```python
from build123d import *

# Parameters (mm, degrees)
ESQUISSE1_R        = 13
BOSS_EXTRU_1_DEPTH = 6.9
ESQUISSE2_R        = 3
BOSS_EXTRU_2_DEPTH = 1
ESQUISSE3_R        = 0.75
BOSS_EXTRU_3_DEPTH = 6
BOSS_EXTRU_4_START = 2.3
ESQUISSE4_R        = 3
BOSS_EXTRU_4_DEPTH = 2.3


with BuildPart() as part:
    # Esquisse1 → Boss.-Extru.1 (new body)
    with BuildSketch(Plane.XY):
        with Locations(Location((0, 0, 0), (0, 0, 180))):
            Circle(ESQUISSE1_R)
    extrude(amount=BOSS_EXTRU_1_DEPTH)

    # Esquisse2 → Boss.-Extru.2 (add)
    with BuildSketch(Plane.XY.offset(6.9)):
        Circle(ESQUISSE2_R)
    extrude(amount=BOSS_EXTRU_2_DEPTH)

    # Esquisse3 → Boss.-Extru.3 (add)
    with BuildSketch(Plane.XY.offset(7.9)):
        Circle(ESQUISSE3_R)
    extrude(amount=BOSS_EXTRU_3_DEPTH)

    # Esquisse4 → Boss.-Extru.4 (add)
    with BuildSketch(Plane(origin=(0, 0, 0), x_dir=(-1, 0, 0), z_dir=(0, 0, -1)).offset(BOSS_EXTRU_4_START)):
        with Locations(Location((0, 0, 0), (0, 0, 180))):
            Circle(ESQUISSE4_R)
    extrude(amount=-BOSS_EXTRU_4_DEPTH)


solid = part.part
```
Work out the finished part from the listing and answer in its coordinate system (mm). A direction names the side the tool comes from. Give positions to 0.01 mm unless a question says otherwise; leave off trailing zeros. Write each loop counter-clockwise with the first axis right and the second up, starting at its lowest first coordinate (ties: lowest second). Pieces come first, ordered by that corner, then holes.
(1) The part is cut by section C-C on z = 10.5. Write down the section's boundary in (x, y), plus the area to 3 significant figures.
Final values:
outline: circle Ø1.5 at (0, 0)
area: 1.77 mm2
(2) Flat-ended cylindrical pins translate along their axes: pin 1 Ø12 at (x, y) = (-1, -8.5) entering from +Z; pin 2 Ø3 at (x, y) = (9, -2.5) entering from -Z; pin 3 Ø3 at (y, z) = (-3.5, 1) entering from -X; pin 4 Ø3 at (x, y) = (0.5, -1) entering from +Z. Find the tip coordinate at first contact, or state that the pin passes through.
Final values:
pin 1: stops at z = 7.9
pin 2: stops at z = 0
pin 3: stops at x = -12.85
pin 4: stops at z = 13.9
(3) The part is cut by section D-D on z = -1. Write down the section's boundary in (x, y).
Final values:
outline: circle Ø6 at (0, 0)
(4) The part is cut by section A-A on x = 0. Write down the section's boundary in (y, z).
Final values:
outline: (-13, 0) - (-3, 0) - (-3, -2.3) - (3, -2.3) - (3, 0) - (13, 0) - (13, 6.9) - (3, 6.9) - (3, 7.9) - (0.75, 7.9) - (0.75, 13.9) - (-0.75, 13.9) - (-0.75, 7.9) - (-3, 7.9) - (-3, 6.9) - (-13, 6.9) - close
(5) The part is cut by section B-B on y = 1.5. Write down the section's boundary in (x, z), plus the area to 3 significant figures.
Final values:
outline: (-12.91, 0) - (-2.6, 0) - (-2.6, -2.3) - (2.6, -2.3) - (2.6, 0) - (12.91, 0) - (12.91, 6.9) - (2.6, 6.9) - (2.6, 7.9) - (-2.6, 7.9) - (-2.6, 6.9) - (-12.91, 6.9) - close
area: 195 mm2
(6) Straight lines are drawn through the part: line 1 (Z direction, x = -6.5, y = 1); line 2 (X direction, y = 11.25, z = 0.5); line 3 (Y direction, x = -7.75, z = 6.5). For each, find the intervals that lie inside material, in ascending order.
Final values:
line 1: z = 0 to 6.9
line 2: x = -6.51 to 6.51
line 3: y = -10.44 to 10.44
(7) Which of the six approach directions +Z, -Z, +X, -X, +Y, -Y give full straight-line access (tool end or side, diameter ignored) to faces 1 (the cylindrical face through (2.86, -0.9, -1.17)), 2 (the cylindrical face through (-3, 0.1, 7.4)), 3 (the cylindrical face through (10.316, 7.91, 3.402))?
Final values:
face 1: -Z
face 2: +Z
face 3: +Z, -Z
